CAD build for the part. Positions are in the model's coordinates, mm. Face numbers are marked on the shaded views. A direction names the side the tool comes from. Round coordinates to 2 decimals unless told otherwise and drop trailing zeros. Loops run counter-clockwise (first coordinate to the right, second up) from the corner with the lowest first, then second, coordinate; pieces in that order, holes last. Notation, with made-up numbers: (-9, 62.5) - (28, 62.5) arc R8 cw to (28, 68.5) - close; hole circle Ø4 at (50.25, 68). An arc over 180 degrees is marked (long way). Use one line per item in the form item = value.
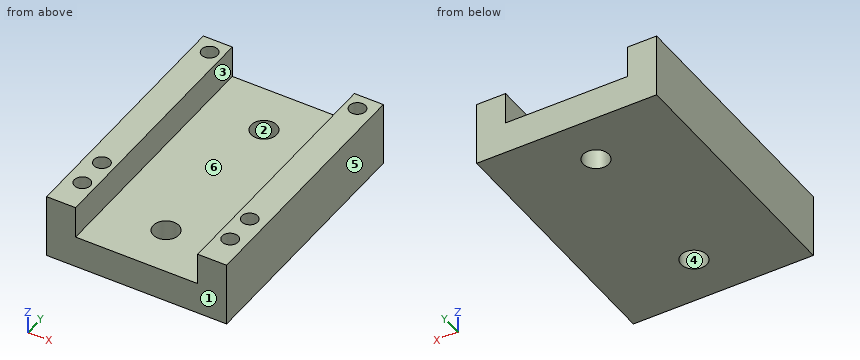
from build123d import *

# Parameters (mm, degrees)
F1_DEPTH = 80
F2_R     = 2.5
F3_DEPTH = 10
F5_D     = 5
F5_DEPTH = 15
F5_TIP   = 1.5021515476
F7_D     = 8


with BuildPart() as f1:
    # F0 (on Front) → F1 (new body)
    with BuildSketch(Plane.XZ):
        Polygon((-19, 20), (-28, 20), (-28, 0), (28, 0), (28, 20), (19, 20), (19, 10), (-19, 10), align=None)
    extrude(amount=F1_DEPTH)

    # F2 (on face) → F3 (cut)
    with BuildSketch(Plane.XY.offset(20)):
        with Locations((23, -60)):
            Circle(F2_R)
        with Locations((-23, -60)):
            Circle(F2_R)
    extrude(amount=-F3_DEPTH, mode=Mode.SUBTRACT)

    # F5
    with Locations(Plane.XY.offset(20)):
        with Locations((-23, -5), (23, -5), (23, -70), (-23, -70)):
            Hole(F5_D / 2, depth=F5_DEPTH)
            with Locations((0, 0, -(F5_DEPTH + F5_TIP / 2))):  # 118° drill point
                Cone(0, F5_D / 2, F5_TIP, mode=Mode.SUBTRACT)

    # F7 (through all)
    with Locations(Plane.XY.offset(10)):
        with Locations((0, -15), (0, -65)):
            Hole(F7_D / 2)


solid = f1.part
1) Tool access for the marked faces 5 and 6: list every direction of +Z, -Z, +X, -X, +Y, -Y with a clear straight run to the whole face (end or side of a thin tool).
Report:
face_5 = +Z, -Z, +X, +Y, -Y
face_6 = +Z, +Y, -Y
2) Drill centre lines: probe 1 along X at (y, z) = (-5, 14.5); probe 2 along Y at (x, z) = (-23, 17); probe 3 along Y at (x, z) = (23, 8.25). Where is each one in solid material? Low to high.
Report:
probe_1 = -28 to -25.5, -20.5 to -19, 19 to 20.5, 25.5 to 28
probe_2 = -80 to -72.5, -67.5 to -62.5, -57.5 to -7.5, -2.5 to 0
probe_3 = -80 to -72.5, -67.5 to -7.5, -2.5 to 0
3) Two-plate mould, pull along Y, no slides. Class the marked faces 1, 2, 3 and 4: +Y half, -Y half, draft (parallel to the pull), parting line (faces both ways), or undercut.
Report:
face_1 = -Y half
face_2 = undercut
face_3 = draft
face_4 = undercut
4) Slice it at C-C (y = -65). Write the cut outline in (x, z), plus the area to 3 significant figures.
Report:
outline = (-28, 0) - (-4, 0) - (-4, 10) - (-19, 10) - (-19, 20) - (-28, 20) - close; (4, 0) - (28, 0) - (28, 20) - (19, 20) - (19, 10) - (4, 10) - close
area = 660 mm^2
5) Slice it at A-A (x = 0). Write the cut outline in (y, z), plus the area to 3 significant figures.
Report:
outline = (-80, 0) - (-69, 0) - (-69, 10) - (-80, 10) - close; (-61, 0) - (-19, 0) - (-19, 10) - (-61, 10) - close; (-11, 0) - (0, 0) - (0, 10) - (-11, 10) - close
area = 640 mm^2
6) Slice it at D-D (z = 15.5). Write the cut outline in (x, y).
Report:
outline = (-28, -80) - (-19, -80) - (-19, 0) - (-28, 0) - close; (19, -80) - (28, -80) - (28, 0) - (19, 0) - close; hole circle Ø5 at (-23, -70); hole circle Ø5 at (-23, -60); hole circle Ø5 at (-23, -5); hole circle Ø5 at (23, -70); hole circle Ø5 at (23, -60); hole circle Ø5 at (23, -5)
7) Flat gauge pins, fed straight in: pin 1 (1 mm diameter, centred on x = 16, y = -57, fed in from +Z); pin 2 (4.5 mm diameter, centred on x = 23, y = -70, fed in from -Z). Where does each tip first touch, or does it go through?
Report:
pin_1 = 10
pin_2 = 0
8) Slice it at B-B (z = 8). Write the cut outline in (x, y), plus the area to 3 significant figures.
Report:
outline = (-28, -80) - (28, -80) - (28, 0) - (-28, 0) - close; hole circle Ø5 at (-23, -70); hole circle Ø5 at (-23, -5); hole circle Ø8 at (0, -65); hole circle Ø8 at (0, -15); hole circle Ø5 at (23, -70); hole circle Ø5 at (23, -5)
area = 4,300 mm^2
